Geometry check sheet. Reference: drawing and pictorial views, mm from the part's lowest x, y, z. A direction names the side the tool comes from. Round coordinates to 2 decimals unless told otherwise and drop trailing zeros. Order: outer loops, then holes, each group sorted by start corner. A loop starts at its lowest first (then second) coordinate and runs counter-clockwise, first axis right, second up.
(1) Release check for a two-part mould opening along X. For the marked faces 3, 4 and 5 record: +X half, -X half, draft (parallel to the pull), parting line (faces both ways), or undercut.
(2) Set-up check for the marked faces 1 and 2: record each of +Z, -Z, +X, -X, +Y, -Y from which the full face is reachable in a straight line by a thin tool's end or side.
(3) Sectioned sample at D-D (x = 47.5). Record the boundary of the cut face in (y, z), plus the area to 3 significant figures.
(4) Sectioned sample at A-A (x = 12.5). Give the number of separate pieces and of enclosed holes in the cut face, plus the area to 3 significant figures.
(5) Sectioned sample at B-B (z = 4.25). Record the boundary of the cut face in (x, y).
(6) Material ranges on line 1 along Y through (x, z) = (41, 4.5); line 2 along X through (y, z) = (18, 5.25); line 3 along Y through (x, z) = (47.5, 2.75), recorded low to high.
(7) Go/stop test with a flat-tipped pin: pin 1 (4 mm diameter, centred on x = 43.5, y = 10, fed in from +Z). Record where the tip stops, or that it passes through.
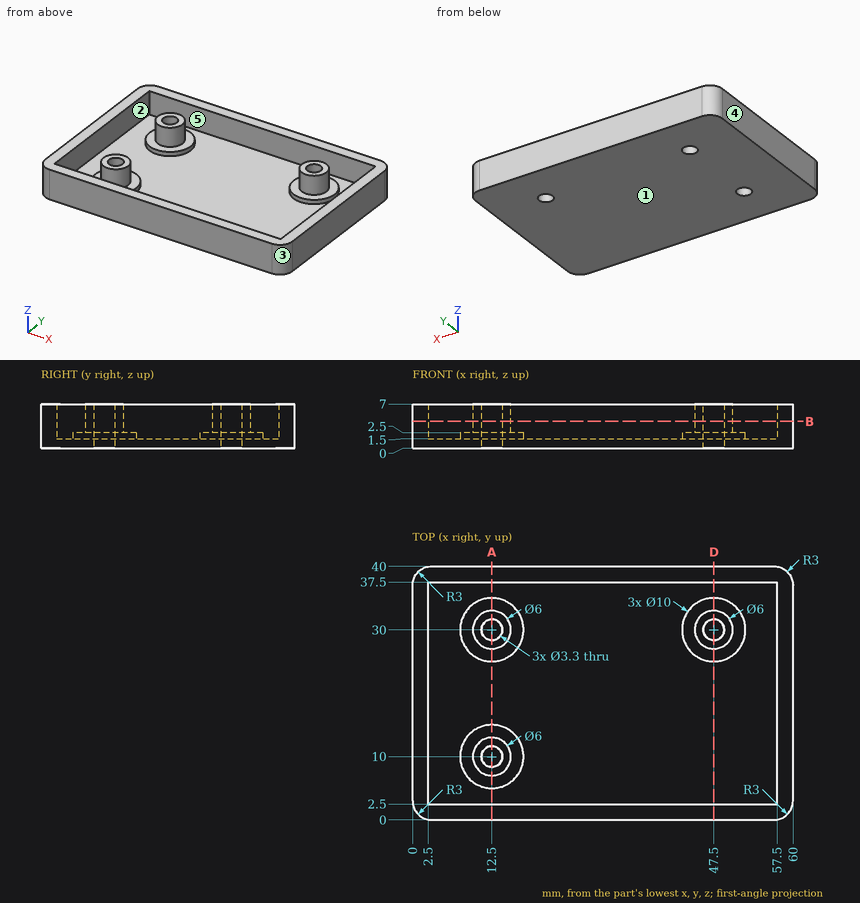
Answer below:
1. face 3: +X half
1. face 4: -X half
1. face 5: undercut
2. face 1: -Z, +X, -X, +Y, -Y
2. face 2: +Z
3. outline: (0, 0) - (28.35, 0) - (28.35, 7) - (27, 7) - (27, 2.5) - (25, 2.5) - (25, 1.5) - (2.5, 1.5) - (2.5, 7) - (0, 7) - close; (31.65, 0) - (40, 0) - (40, 7) - (37.5, 7) - (37.5, 1.5) - (35, 1.5) - (35, 2.5) - (33, 2.5) - (33, 7) - (31.65, 7) - close
3. area: 101 mm2
4. separate pieces: 3
4. enclosed holes: 0
4. area: 115 mm2
5. outline: (0, 3) arc R3 ccw to (3, 0) - (57, 0) arc R3 ccw to (60, 3) - (60, 37) arc R3 ccw to (57, 40) - (3, 40) arc R3 ccw to (0, 37) - close; circle Ø6 at (12.5, 10); circle Ø6 at (12.5, 30); circle Ø6 at (47.5, 30); hole (2.5, 2.5) - (57.5, 2.5) - (57.5, 37.5) - (2.5, 37.5) - close; hole circle Ø3.3 at (12.5, 10); hole circle Ø3.3 at (12.5, 30); hole circle Ø3.3 at (47.5, 30)
6. line 1: y = 0 to 2.5, 37.5 to 40
6. line 2: x = 0 to 2.5, 57.5 to 60
6. line 3: y = 0 to 2.5, 27 to 28.35, 31.65 to 33, 37.5 to 40
7. pin 1: stops at z = 1.5
